Answer from the drawing. Dimensions are ordinates in mm from the lowest x, y and z of the part. Give positions to 0.01 mm unless a question says otherwise; leave off trailing zeros. Loops run counter-clockwise (first coordinate to the right, second up) from the corner with the lowest first, then second, coordinate; pieces in that order, holes last. Notation, with made-up numbers: (25, 73.25) -> (44, 73.25) arc R17 cw to (44, 102.25) -> close; hole circle Ø9 at (71.25, 45.25). An arc over 180 degrees is marked (long way). Write each question's results on one line, items separated by ' | '. Start each with the question number.
Item 1: Each of these flat-tipped pins is pushed along its axis until it touches: P1, Ø1.5, axis at y = 3.5, z = 61, coming from the +X side; P2, Ø2.5, axis at y = 3, z = 6, coming from the +X side; P3, Ø4.5, axis at x = 246.5, y = 6, coming from the -Z side. Where does it stop, or does it pass through?
Item 2: Section A-A on y = 2.5 is taken. Write down the section's boundary in (x, z).
Item 3: Find the intervals of material crossed by line 1 (X direction, y = 1.5, z = 5); line 2 (Z direction, x = 160, y = 3); line 3 (X direction, y = 2.5, z = 55.5), in increasing order.
Item 4: Section B-B on x = 225 is taken. Write down the section's boundary in (y, z).
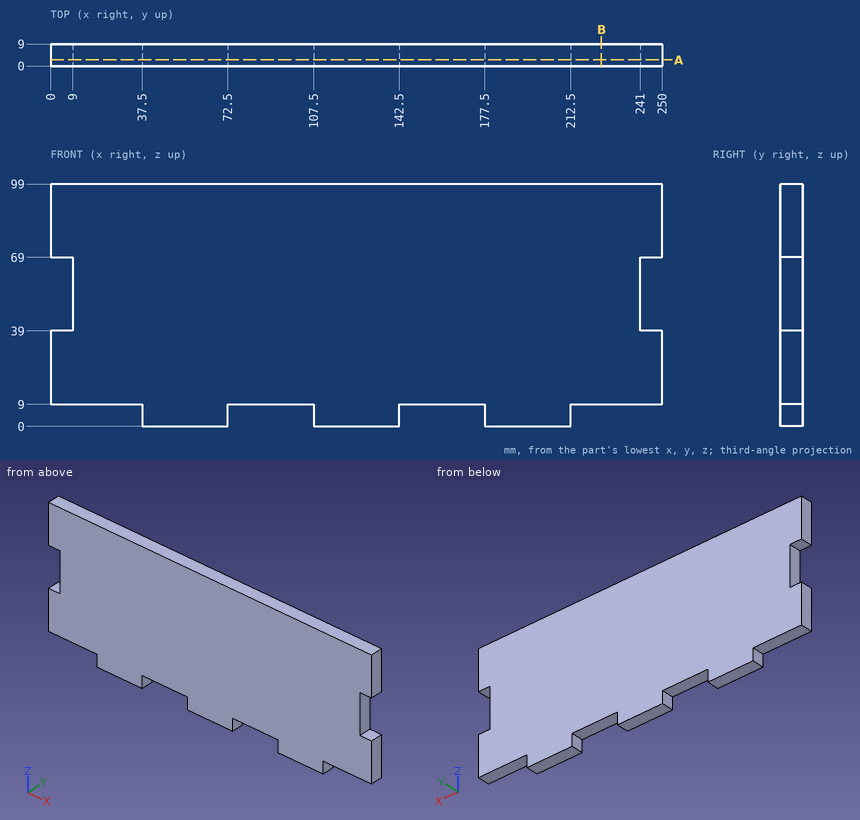
Findings:
1) P1: x = 241 | P2: x = 212.5 | P3: z = 9
2) outline: (0, 9) -> (37.5, 9) -> (37.5, 0) -> (72.5, 0) -> (72.5, 9) -> (107.5, 9) -> (107.5, 0) -> (142.5, 0) -> (142.5, 9) -> (177.5, 9) -> (177.5, 0) -> (212.5, 0) -> (212.5, 9) -> (250, 9) -> (250, 39) -> (241, 39) -> (241, 69) -> (250, 69) -> (250, 99) -> (0, 99) -> (0, 69) -> (9, 69) -> (9, 39) -> (0, 39) -> close
3) line 1: 37.5 to 72.5, 107.5 to 142.5, 177.5 to 212.5 | line 2: 9 to 99 | line 3: 9 to 241
4) outline: (0, 9) -> (9, 9) -> (9, 99) -> (0, 99) -> close
